```python
from build123d import *

# Parameters (mm, degrees)
F0_W     = 482.6
F0_H     = 389.636
F1_DEPTH = 19.304
F2_D     = 355.6
F3_W     = 19.304
F3_H     = 19.304
F3_W_2   = 443.992
F3_H_2   = 351.028
F4_DEPTH = 6.35


with BuildPart() as f1:
    # F0 (on Top) → F1 (new body)
    with BuildSketch(Plane.XY):
        Rectangle(F0_W, F0_H)
    extrude(amount=F1_DEPTH)

    # F2 (through all)
    with Locations(Plane(origin=(0, 0, 0), x_dir=(1, 0, 0), z_dir=(0, 0, -1))):
        with Locations((0, 0)):
            Hole(F2_D / 2)

    # F3 (on face) → F4 (cut)
    with BuildSketch(Plane.XY.offset(19.304)):
        with Locations((-231.648, 185.166)):
            Rectangle(F3_W, F3_H)
        with Locations((0, 185.166)):
            Rectangle(F3_W_2, F3_H)
        with Locations((-231.648, 0)):
            Rectangle(F3_W, F3_H_2)
        with Locations((231.648, 185.166)):
            Rectangle(F3_W, F3_H)
        with Locations((-231.648, -185.166)):
            Rectangle(F3_W, F3_H)
        with Locations((231.648, 0)):
            Rectangle(F3_W, F3_H_2)
        with Locations((0, -185.166)):
            Rectangle(F3_W_2, F3_H)
        with Locations((231.648, -185.166)):
            Rectangle(F3_W, F3_H)
    extrude(amount=-F4_DEPTH, mode=Mode.SUBTRACT)


solid = f1.part
```
CAD build for the part. Positions are in the model's coordinates, mm. Round coordinates to 2 decimals unless told otherwise and drop trailing zeros. Write each loop counter-clockwise with the first axis right and the second up, starting at its lowest first coordinate (ties: lowest second). Pieces come first, ordered by that corner, then holes. Notation, with made-up numbers: M 53.5,14 L 59.5,14 A18 ccw 59.5,23 Z; hole C 7.25,23.5 d7. An arc over 180 degrees is marked long. One line per question, with ' | ' between items.
1. Mould opens along X. For faces 1 (the flat face through (188, 2, 19.304)), 2 (the cylindrical face through (38.544, 173.572, 9.787)), 3 (the flat face through (-241.3, -3, 6)) say: pulls with the +X half, pulls with the -X half, needs draft (parallel to the pull), parting line crosses it, or undercut.
Working result:
face 1: needs draft | face 2: undercut | face 3: pulls with the -X half
2. Cut at A-A on y = 0. Write the cut outline in (x, z), and give its area (3 significant figures).
Working result:
outline: M -241.3,0 L -177.8,0 L -177.8,19.3 L -222,19.3 L -222,12.95 L -241.3,12.95 Z; M 177.8,0 L 241.3,0 L 241.3,12.95 L 222,12.95 L 222,19.3 L 177.8,19.3 Z | area: 2,210 mm2
3. Cut at D-D on x = -201. Write the cut outline in (y, z), and give its area (3 significant figures).
Working result:
outline: M -194.82,0 L 194.82,0 L 194.82,12.95 L 175.51,12.95 L 175.51,19.3 L -175.51,19.3 L -175.51,12.95 L -194.82,12.95 Z | area: 7,280 mm2
4. Cut at C-C on z = 6. Write the cut outline in (x, y).
Working result:
outline: M -241.3,-194.82 L 241.3,-194.82 L 241.3,194.82 L -241.3,194.82 Z; hole C 0,0 d355.6
5. Cut at B-B on x = 0. Write the cut outline in (y, z), and give its area (3 significant figures).
Working result:
outline: M -194.82,0 L -177.8,0 L -177.8,12.95 L -194.82,12.95 Z; M 177.8,0 L 194.82,0 L 194.82,12.95 L 177.8,12.95 Z | area: 441 mm2
6. Pin check, flat tips, straight feed: pin 1 Ø3 at (y, z) = (-123, 14.5) entering from -X; pin 2 Ø5 at (x, z) = (127.5, 17) entering from +Y; pin 3 Ø3 at (x, z) = (-122, 17.5) entering from -Y; pin 4 Ø7 at (x, z) = (-141, 15.5) entering from +Y. Stop position of each tip, or through.
Working result:
pin 1: x = -222 | pin 2: y = 175.51 | pin 3: y = -175.51 | pin 4: y = 194.82
7. Probe L1, parallel to Y at x = 0, z = 5.25; L2, parallel to X at y = 29, z = 18; L3, parallel to X at y = 90, z = 4.5. List the from-to ranges inside material, lowest first. Write a range as from..to.
Working result:
L1: -194.82..-177.8, 177.8..194.82 | L2: -222..-175.42, 175.42..222 | L3: -241.3..-153.34, 153.34..241.3
